Build history of the part. All positions in model axes, mm. A direction names the side the tool comes from. Round coordinates to 2 decimals unless told otherwise and drop trailing zeros. Write each loop counter-clockwise with the first axis right and the second up, starting at its lowest first coordinate (ties: lowest second). Pieces come first, ordered by that corner, then holes. Notation, with made-up numbers: (58.5, -30) - (70.5, -30) arc R18 cw to (70.5, 3) - close; hole circle Ø1 at (-12, -27.75). An arc over 180 degrees is marked (long way). One line per question, with ' | ' between items.
from build123d import *

# Parameters (mm, degrees)
SKETCH_1_W          = 21
SKETCH_1_H          = 21
SKETCH_1_R          = 4
EXTRUDE_1_DEPTH     = 3.5
SKETCH_2_R          = 2.25
SKETCH_2_R_2        = 1.5
CUT_EXTRUDE_1_DEPTH = 1.5
SKETCH_2_2_R        = 1.5
CUT_EXTRUDE_2_DEPTH = 16.256146302
SKETCH_4_R          = 2.55
CUT_EXTRUDE_3_DEPTH = 16.256146302
EXTRUDE_2_DEPTH     = 3.5
SKETCH_6_W          = 26.9
SKETCH_6_H          = 2
EXTRUDE_3_DEPTH     = 3.5


with BuildPart() as part:
    # 草图1 → 凸台-拉伸1 (new body)
    with BuildSketch(Plane(origin=(0, 0, 0), x_dir=(0, 0, -1), z_dir=(1, 0, 0))):
        Rectangle(SKETCH_1_W, SKETCH_1_H)
        Circle(SKETCH_1_R, mode=Mode.SUBTRACT)
    extrude(amount=EXTRUDE_1_DEPTH)

    # 草图2 → 切除-拉伸1 (cut)
    # profile 1 of 2: a face of its own
    with BuildSketch(Plane.ZY):
        with Locations((0, 7.2)):
            Circle(SKETCH_2_R)
        with Locations((0, 7.2)):
            Circle(SKETCH_2_R_2, mode=Mode.SUBTRACT)
    # profile 2 of 2: a face of its own
    with BuildSketch(Plane.ZY):
        with Locations((0, -7.2)):
            Circle(SKETCH_2_R)
        with Locations((0, -7.2)):
            Circle(SKETCH_2_R_2, mode=Mode.SUBTRACT)
    extrude(amount=-CUT_EXTRUDE_1_DEPTH, mode=Mode.SUBTRACT)

    # 草图2<2> → 切除-拉伸2 (cut, through all)
    with BuildSketch(Plane.ZY):
        with Locations((0, 7.2)):
            Circle(SKETCH_2_2_R)
        with Locations((0, -7.2)):
            Circle(SKETCH_2_2_R)
    extrude(amount=-CUT_EXTRUDE_2_DEPTH, mode=Mode.SUBTRACT)

    # 草图4 → 切除-拉伸3 (cut, through all)
    with BuildSketch(Plane.ZY):
        with Locations((-5.590169944, 5)):
            Circle(SKETCH_4_R)
    extrude(amount=-CUT_EXTRUDE_3_DEPTH, mode=Mode.SUBTRACT)

    # 草图5 → 凸台-拉伸2 (add)
    with BuildSketch(Plane.ZY):
        with BuildLine():
            Line((-10.5, -10.5), (-10.5, 10.5))
            Line((-10.5, 10.5), (-16.4, 10.5))
            Line((-16.4, 10.5), (-16.4, 2.934341014))
            Line((-16.4, 2.934341014), (-13.090169944, 2.934341014))
            ThreePointArc((-13.090169944, 2.934341014), (-11.852733077, 2.421777882), (-11.340169944, 1.184341014))
            ThreePointArc((-11.340169944, 1.184341014), (-11.852733077, -0.053095853), (-13.090169944, -0.565658986))
            Line((-13.090169944, -0.565658986), (-16.4, -0.565658986))
            Line((-16.4, -0.565658986), (-16.4, -10.5))
            Line((-16.4, -10.5), (-10.5, -10.5))
        make_face()
    extrude(amount=-EXTRUDE_2_DEPTH)

    # 草图6 → 凸台-拉伸3 (add)
    with BuildSketch(Plane.ZY):
        with Locations((-2.95, 11.5)):
            Rectangle(SKETCH_6_W, SKETCH_6_H)
    extrude(amount=-EXTRUDE_3_DEPTH)


solid = part.part
Q1. Saw through at C-C, the plane z = 0. List the corners of the cut face in (x, y), then the cut area to 3 significant figures.
Found:
outline: (0, -10.5) - (3.5, -10.5) - (3.5, -8.7) - (1.5, -8.7) - (1.5, -9.45) - (0, -9.45) - close; (0, -4.95) - (1.5, -4.95) - (1.5, -5.7) - (3.5, -5.7) - (3.5, -4) - (0, -4) - close; (0, 4) - (3.5, 4) - (3.5, 5.7) - (1.5, 5.7) - (1.5, 4.95) - (0, 4.95) - close; (0, 9.45) - (1.5, 9.45) - (1.5, 8.7) - (3.5, 8.7) - (3.5, 12.5) - (0, 12.5) - close | area: 27.0 mm^2
Q2. Pull direction Y, two halves, no side cores. Call faces 4 (the flat face through (2, 8, -16.4)), 5 (the flat face through (2, -0.566, -15)), 6 (the flat face through (2, 12.5, -3)): +Y half, -Y half, draft (parallel to the pull), parting line (faces both ways), or undercut.
Found:
face 4: draft | face 5: undercut | face 6: +Y half
Q3. Saw through at D-D, the plane z = -12. List the corners of the cut face in (x, y), then the cut area to 3 significant figures.
Found:
outline: (0, -10.5) - (3.5, -10.5) - (3.5, -0.18) - (0, -0.18) - close; (0, 2.55) - (3.5, 2.55) - (3.5, 12.5) - (0, 12.5) - close | area: 70.9 mm^2
Q4. Saw through at A-A, the plane y = -7.2. List the corners of the cut face in (x, z).
Found:
outline: (0, -16.4) - (3.5, -16.4) - (3.5, -1.5) - (1.5, -1.5) - (1.5, -2.25) - (0, -2.25) - close; (0, 2.25) - (1.5, 2.25) - (1.5, 1.5) - (3.5, 1.5) - (3.5, 10.5) - (0, 10.5) - close
Q5. Which spindle directions (+Z, -Z, +X, -X, +Y, -Y) get a long thin tool onto all of the face, cutting with end or side? Do faces 1 (the cylindrical face through (2.486, 5.736, -0.325)), 2 (the flat face through (1.5, 9, 0)), 3 (the flat face through (2, 2.934, -15)). Say none if no direction does.
Found:
face 1: +X, -X | face 2: -X | face 3: -Z, +X, -X
Q6. Drill centre lines: L1, parallel to Y at x = 0.55, z = 0; L2, parallel to Y at x = 2.2, z = -14.25; L3, parallel to Y at x = 3.25, z = 1. Where is each one in solid material? Low to high. Write a range as from..to.
Found:
L1: -10.5..-9.45, -4.95..-4, 4..4.95, 9.45..12.5 | L2: -10.5..-0.57, 2.93..12.5 | L3: -10.5..-8.32, -6.08..-3.87, 3.87..6.08, 8.32..12.5
Q7. Saw through at B-B, the plane x = 2.2. List the corners of the cut face in (y, z), then the cut area to 3 significant figures.
Found:
outline: (-10.5, -16.4) - (-0.57, -16.4) - (-0.57, -13.09) arc R1.75 cw to (2.93, -13.09) - (2.93, -16.4) - (12.5, -16.4) - (12.5, 10.5) - (-10.5, 10.5) - close; hole circle Ø3 at (-7.2, 0); hole circle Ø8 at (0, 0); hole circle Ø5.1 at (5, -5.59); hole circle Ø3 at (7.2, 0) | area: 517 mm^2
